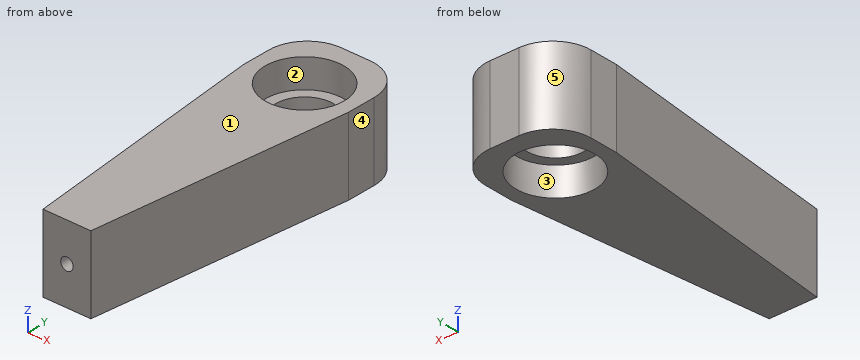
```python
from build123d import *

# Parameters (mm, degrees)
SKETCH_1_W          = 11
SKETCH_1_H          = 8
EXTRUDE_1_DEPTH     = 34
SKETCH_2_R          = 4.1
CUT_EXTRUDE_1_DEPTH = 3
SKETCH_4_R          = 3
CUT_EXTRUDE_3_DEPTH = 6
SKETCH_6_OUTSIDE_W  = 20.324
SKETCH_6_OUTSIDE_H  = 43.324
CUT_EXTRUDE_5_DEPTH = 10
FILLET_1_R          = 4
SKETCH_5_R          = 0.65
CUT_EXTRUDE_4_DEPTH = 20
SKETCH_7_R          = 4.1
CUT_EXTRUDE_6_DEPTH = 3


with BuildPart() as part:
    # Эскиз1 → Бобышка-Вытянуть1 (new body)
    with BuildSketch(Plane(origin=(0, 0, 0), x_dir=(1, 0, 0), z_dir=(0, 1, 0))):
        Rectangle(SKETCH_1_W, SKETCH_1_H)
    extrude(amount=EXTRUDE_1_DEPTH)

    # Эскиз2 → Вырез-Вытянуть1 (cut)
    with BuildSketch(Plane(origin=(0, 0, -4), x_dir=(-1, 0, 0), z_dir=(0, 0, -1))):
        with Locations((0, 28)):
            Circle(SKETCH_2_R)
    extrude(amount=-CUT_EXTRUDE_1_DEPTH, mode=Mode.SUBTRACT)

    # Эскиз4 → Вырез-Вытянуть3 (cut, through all)
    with BuildSketch(Plane(origin=(0, 0, -1), x_dir=(-1, 0, 0), z_dir=(0, 0, -1))):
        with Locations((0, 28)):
            Circle(SKETCH_4_R)
    extrude(amount=-CUT_EXTRUDE_3_DEPTH, mode=Mode.SUBTRACT)

    # Эскиз6 outside → Вырез-Вытянуть5 (cut)
    with BuildSketch(Plane(origin=(0, 0, -4), x_dir=(-1, 0, 0), z_dir=(0, 0, -1))):
        with Locations((0, 17)):
            Rectangle(SKETCH_6_OUTSIDE_W, SKETCH_6_OUTSIDE_H)
        Polygon((-5.5, 27), (-2.5, 0), (2.5, 0), (5.5, 27), (5.5, 34), (-5.5, 34), align=None, mode=Mode.SUBTRACT)
    extrude(amount=-CUT_EXTRUDE_5_DEPTH, mode=Mode.SUBTRACT)

    # Скругление1
    fillet_1_edges = [part.edges().sort_by_distance(p)[0] for p in [
        (5.5, 34, 0),
        (-5.5, 34, 0),
    ]]
    fillet(fillet_1_edges, radius=FILLET_1_R)

    # Эскиз5 → Вырез-Вытянуть4 (cut)
    with BuildSketch(Plane.XZ):
        Circle(SKETCH_5_R)
    extrude(amount=-CUT_EXTRUDE_4_DEPTH, mode=Mode.SUBTRACT)

    # Эскиз7 → Вырез-Вытянуть6 (cut)
    with BuildSketch(Plane.XY.offset(4)):
        with Locations((0, 28)):
            Circle(SKETCH_7_R)
    extrude(amount=-CUT_EXTRUDE_6_DEPTH, mode=Mode.SUBTRACT)


solid = part.part
```
Work out the finished part from the listing and answer in its coordinate system (mm). Face numbers are marked on the shaded views. A direction names the side the tool comes from. Round coordinates to 2 decimals unless told otherwise and drop trailing zeros. Loops run counter-clockwise (first coordinate to the right, second up) from the corner with the lowest first, then second, coordinate; pieces in that order, holes last.
(1) Each of these flat-tipped pins is pushed along its axis until it touches: P1, Ø3, axis at y = 16, z = 1.5, coming from the +X side; P2, Ø4, axis at y = 21, z = -1.5, coming from the -X side; P3, Ø5, axis at x = 0, y = 28, coming from the -Z side; P4, Ø4, axis at x = 1, y = 26.5, coming from the -Z side. Where does it stop, or does it pass through?
Computed values:
P1: stops at x = 4.44
P2: stops at x = -5.06
P3: passes through
P4: stops at z = -1
(2) The part is cut by section D-D, the plane y = 10.5. Give the vertices of the cut face in (x, z), and give its area (3 significant figures).
Computed values:
outline: (-3.67, -4) - (3.67, -4) - (3.67, 4) - (-3.67, 4) - close; hole circle Ø1.3 at (0, 0)
area: 57.3 mm2
(3) For the marked faces 1 and 2, determine the directions among +Z, -Z, +X, -X, +Y, -Y from which every point of the face is accessible in a straight line to the end or side of a thin tool.
Computed values:
face 1: +Z, +X, -X, +Y, -Y
face 2: +Z
(4) The part is cut by section B-B, the plane x = 0. Give the vertices of the cut face in (y, z).
Computed values:
outline: (0, -4) - (23.9, -4) - (23.9, -1) - (25, -1) - (25, 1) - (23.9, 1) - (23.9, 4) - (0, 4) - (0, 0.65) - (20, 0.65) - (20, -0.65) - (0, -0.65) - close; (31, -1) - (32.1, -1) - (32.1, -4) - (34, -4) - (34, 4) - (32.1, 4) - (32.1, 1) - (31, 1) - close
(5) Find the intervals of material crossed by L1, parallel to Y at x = 0, z = -1.7; L2, parallel to X at y = 17, z = -0.25; L3, parallel to X at y = 25, z = 1.75, in increasing order.
Computed values:
L1: y = 0 to 23.9, 32.1 to 34
L2: x = -4.39 to -0.6, 0.6 to 4.39
L3: x = -5.28 to -2.79, 2.79 to 5.28
(6) The part is cut by section C-C, the plane z = -3. Give the vertices of the cut face in (x, y), and give its area (3 significant figures).
Computed values:
outline: (-5.5, 27) - (-2.5, 0) - (2.5, 0) - (5.5, 27) - (5.5, 30) arc R4 ccw to (1.5, 34) - (-1.5, 34) arc R4 ccw to (-5.5, 30) - close; hole circle Ø8.2 at (0, 28)
area: 233 mm2
(7) The part is cut by section A-A, the plane y = 28. Give the vertices of the cut face in (x, z), and give its area (3 significant figures).
Computed values:
outline: (-5.5, -4) - (-4.1, -4) - (-4.1, -1) - (-3, -1) - (-3, 1) - (-4.1, 1) - (-4.1, 4) - (-5.5, 4) - close; (3, -1) - (4.1, -1) - (4.1, -4) - (5.5, -4) - (5.5, 4) - (4.1, 4) - (4.1, 1) - (3, 1) - close
area: 26.8 mm2
(8) The mould has two halves that part along Y. Classify the marked faces 3, 4 and 5: pulls with the +Y half, pulls with the -Y half, needs draft (parallel to the pull), parting line crosses it, or undercut.
Computed values:
face 3: undercut
face 4: needs draft
face 5: pulls with the +Y half
